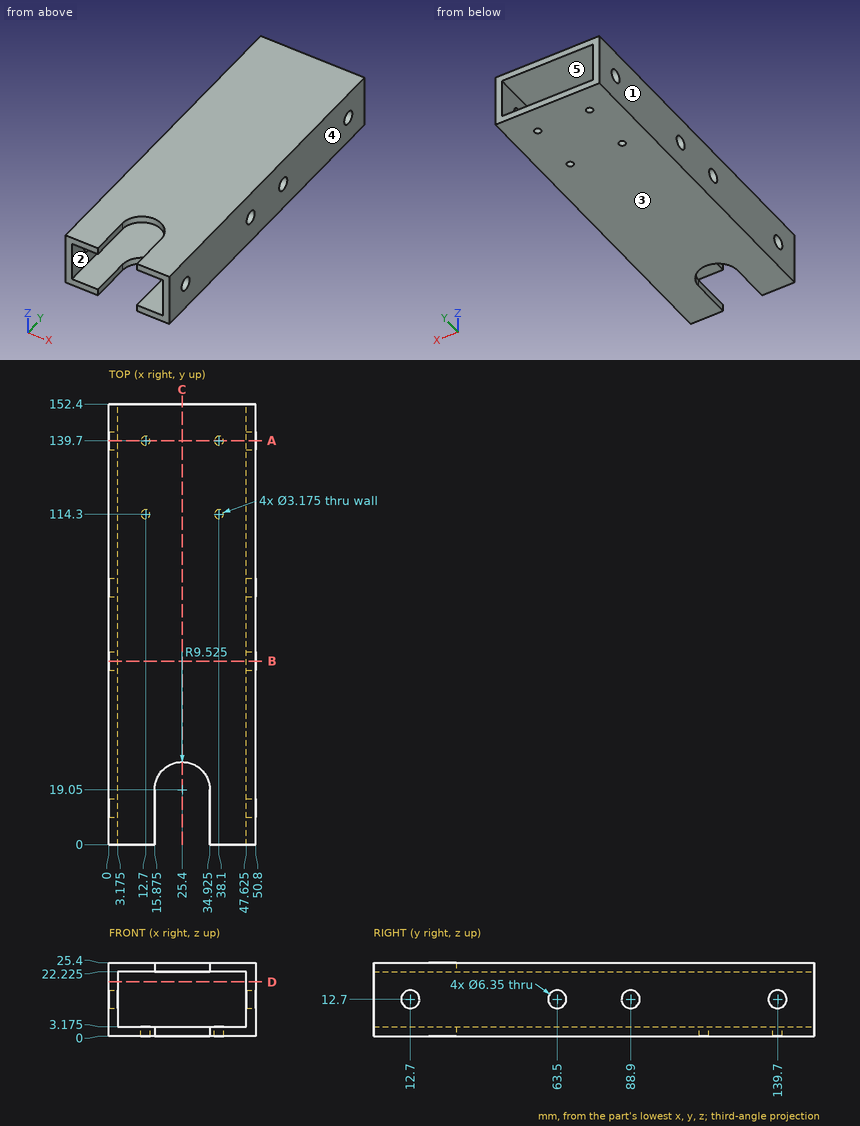
Print and shaded views of the part. All mm, measured from the part's lowest x, y and z. A direction names the side the tool comes from. Round coordinates to 2 decimals unless told otherwise and drop trailing zeros. Write each loop counter-clockwise with the first axis right and the second up, starting at its lowest first coordinate (ties: lowest second). Pieces come first, ordered by that corner, then holes. Notation, with made-up numbers: (36, 24) - (91, 24) arc R33 cw to (91, 53) - close; hole circle Ø10 at (-15.75, 67.25). An arc over 180 degrees is marked (long way). One line per question, with ' | ' between items.
1. Band-saw the part on B-B, the plane y = 63.5. Write the cut outline in (x, z) (3 decimals).
Results are:
outline: (0, 0) - (50.8, 0) - (50.8, 9.525) - (47.625, 9.525) - (47.625, 3.175) - (3.175, 3.175) - (3.175, 9.525) - (0, 9.525) - close; (0, 15.875) - (3.175, 15.875) - (3.175, 22.225) - (47.625, 22.225) - (47.625, 15.875) - (50.8, 15.875) - (50.8, 25.4) - (0, 25.4) - close
2. Band-saw the part on A-A, the plane y = 139.7. Write the cut outline in (x, z) (1 decimal), and give its area (3 significant figures).
Results are:
outline: (0, 0) - (11.1, 0) - (11.1, 3.2) - (3.2, 3.2) - (3.2, 9.5) - (0, 9.5) - close; (0, 15.9) - (3.2, 15.9) - (3.2, 22.2) - (47.6, 22.2) - (47.6, 15.9) - (50.8, 15.9) - (50.8, 25.4) - (0, 25.4) - close; (14.3, 0) - (36.5, 0) - (36.5, 3.2) - (14.3, 3.2) - close; (39.7, 0) - (50.8, 0) - (50.8, 9.5) - (47.6, 9.5) - (47.6, 3.2) - (39.7, 3.2) - close | area: 383 mm^2
3. Drop flat-ended pins along their axis: pin 1 Ø5 at (x, z) = (44, 17) entering from +Y; pin 2 Ø2.5 at (x, y) = (12.7, 139.7) entering from -Z (3 decimals). Give the stop position or say it passes through.
Results are:
pin 1: through | pin 2: z = 22.225
4. Tool access for the marked faces 4 and 5: list every direction of +Z, -Z, +X, -X, +Y, -Y with a clear straight run to the whole face (end or side of a thin tool).
Results are:
face 4: +Z, -Z, +X, +Y, -Y | face 5: +Y, -Y
5. Mould opens along Z. For the marked faces 1, 2 and 3 say: released by +Z, released by -Z, zero draft, split by the parting line, or undercut.
Results are:
face 1: zero draft | face 2: undercut | face 3: released by -Z
6. Band-saw the part on C-C, the plane x = 25.4. Write the cut outline in (y, z) (3 decimals), and give its area (3 significant figures).
Results are:
outline: (28.575, 0) - (152.4, 0) - (152.4, 3.175) - (28.575, 3.175) - close; (28.575, 22.225) - (152.4, 22.225) - (152.4, 25.4) - (28.575, 25.4) - close | area: 786 mm^2
7. Band-saw the part on D-D, the plane z = 18.75. Write the cut outline in (x, y) (3 decimals), and give its area (3 significant figures).
Results are:
outline: (0, 0) - (3.175, 0) - (3.175, 152.4) - (0, 152.4) - close; (47.625, 0) - (50.8, 0) - (50.8, 152.4) - (47.625, 152.4) - close | area: 968 mm^2
8. Drill centre lines: line 1 along X through (y, z) = (114.3, 2.1); line 2 along Y through (x, z) = (48.7, 12.7) (3 decimals); line 3 along Z through (x, y) = (47, 13.5) (3 decimals). Where is each one in solid material? Low to high. Write a range as from..to.
Results are:
line 1: 0..11.11, 14.29..36.51, 39.69..50.8 | line 2: 0..9.525, 15.875..60.325, 66.675..85.725, 92.075..136.525, 142.875..152.4 | line 3: 0..3.175, 22.225..25.4
